from build123d import *

# Parameters (mm, degrees)
F0_W     = 7.7
F0_H     = 7.7
F0_W_2   = 5
F0_H_2   = 5
F1_DEPTH = 4.6
F2_R     = 0.5
F3_R     = 0.5


with BuildPart() as f1:
    # F0 (on Front) → F1 (new body)
    with BuildSketch(Plane.XZ):
        Rectangle(F0_W, F0_H)
        Rectangle(F0_W_2, F0_H_2, mode=Mode.SUBTRACT)
    extrude(amount=F1_DEPTH)

    # F2
    f2_edges = [f1.edges().sort_by_distance(p)[0] for p in [
        (2.5, -2.3, 2.5),
        (-2.5, -2.3, 2.5),
        (2.5, -2.3, -2.5),
        (-2.5, -2.3, -2.5),
    ]]
    fillet(f2_edges, radius=F2_R)

    # F3
    f3_edges = [f1.edges().sort_by_distance(p)[0] for p in [
        (3.85, -2.3, 3.85),
        (3.85, -2.3, -3.85),
        (-3.85, -2.3, -3.85),
        (-3.85, -2.3, 3.85),
    ]]
    fillet(f3_edges, radius=F3_R)


solid = f1.part
Design review of the part built by this model. Coordinates are the model's own, in mm. A direction names the side the tool comes from. Coordinates: 2 decimals unless noted, no trailing zeros. Order: outer loops, then holes, each group sorted by start corner. A loop starts at its lowest first (then second) coordinate and runs counter-clockwise, first axis right, second up. Notation, with made-up numbers: (-39, 10) -> (-14, 10) arc R10 ccw to (-14, 19) -> close; hole circle Ø3 at (-35, 60). An arc over 180 degrees is marked (long way). One line per item, written item: value.
1) We need section A-A, the plane x = 1.75. Give the boundary of the cut face in (y, z).
Output values:
outline: (-4.6, -3.85) -> (0, -3.85) -> (0, -2.5) -> (-4.6, -2.5) -> close; (-4.6, 2.5) -> (0, 2.5) -> (0, 3.85) -> (-4.6, 3.85) -> close
2) Draft analysis for pull direction X (two halves, no side actions). For faces 3 (the face through (0, -2, -3.85)), 4 (the face through (-3.85, -2, 0)), 5 (the face through (2.5, -2, 0)), state which applies: +X half, -X half, draft (parallel to the pull), parting line (faces both ways), or undercut.
Output values:
face 3: draft
face 4: -X half
face 5: undercut
3) Machinability: for faces 1 (the face through (-3, -4.6, 0)), 2 (the face through (-2.5, -2, 0)), which of the approach directions +Z, -Z, +X, -X, +Y, -Y give a long, thin tool a straight path to every point of the face, cutting with its end or side? Answer none if there is none.
Output values:
face 1: +Z, -Z, +X, -X, -Y
face 2: +Y, -Y
4) To check wall thickness, follow probe 1 along X at (y, z) = (-0.95, 1.5); probe 2 along Z at (x, y) = (-2.25, -1.35). State the ranges of each line that lie inside material, in increasing order. Write a range as [from, to].
Output values:
probe 1: x = [-3.85, -2.5], [2.5, 3.85]
probe 2: z = [-3.85, -2.43], [2.43, 3.85]
5) We need section C-C, the plane z = 1.25. Give the boundary of the cut face in (x, y).
Output values:
outline: (-3.85, -4.6) -> (-2.5, -4.6) -> (-2.5, 0) -> (-3.85, 0) -> close; (2.5, -4.6) -> (3.85, -4.6) -> (3.85, 0) -> (2.5, 0) -> close
6) We need section B-B, the plane y = -0.3. Give the boundary of the cut face in (x, z).
Output values:
outline: (-3.85, -3.35) arc R0.5 ccw to (-3.35, -3.85) -> (3.35, -3.85) arc R0.5 ccw to (3.85, -3.35) -> (3.85, 3.35) arc R0.5 ccw to (3.35, 3.85) -> (-3.35, 3.85) arc R0.5 ccw to (-3.85, 3.35) -> close; hole (-2.5, -2) arc R0.5 ccw to (-2, -2.5) -> (2, -2.5) arc R0.5 ccw to (2.5, -2) -> (2.5, 2) arc R0.5 ccw to (2, 2.5) -> (-2, 2.5) arc R0.5 ccw to (-2.5, 2) -> close
